from build123d import *

# Parameters (mm, degrees)
F0_W     = 11.5173384978
F0_H     = 13.0775373821
F0_W_2   = 16.1038693041
F0_H_2   = 2.9893541513
F1_DEPTH = 3


with BuildPart() as f1:
    # F0 (on Top) → F1 (new body)
    with BuildSketch(Plane.XY):
        with BuildLine():
            Line((-27.644963935, 33.9523106813), (-20.6479323776, 25.2299834391))
            ThreePointArc((-20.6479323776, 25.2299834391), (-19.752349447, 27.8264836408), (-19.4488823526, 30.5562803009))
            ThreePointArc((-19.4488823526, 30.5562803009), (-41.5954351034, 38.3068214365), (-29.1147480721, 18.4379226783))
            Line((-29.1147480721, 18.4379226783), (-36.1117796295, 27.1602499205))
            Line((-36.1117796295, 27.1602499205), (-27.644963935, 33.9523106813))
        make_face()
        with BuildLine():
            ThreePointArc((-29.1147480721, 18.4379226783), (-24.1007453474, 20.8608827061), (-20.6479323776, 25.2299834391))
            Line((-20.6479323776, 25.2299834391), (-27.644963935, 33.9523106813))
            Line((-27.644963935, 33.9523106813), (-36.1117796295, 27.1602499205))
            Line((-36.1117796295, 27.1602499205), (-29.1147480721, 18.4379226783))
        make_face()
        with BuildLine():
            Line((-19.5692731498, 6.5387686911), (-8.051934652, 9.5281228423))
            Line((-8.051934652, 9.5281228423), (-20.6479323776, 25.2299834391))
            ThreePointArc((-20.6479323776, 25.2299834391), (-24.1007453474, 20.8608827061), (-29.1147480721, 18.4379226783))
            Line((-29.1147480721, 18.4379226783), (-19.5692731498, 6.5387686911))
        make_face()
        with BuildLine():
            ThreePointArc((44.3078612119, 30.5562803009), (29.1485751221, 42.6823026363), (20.6479323776, 25.2299834391))
            Line((20.6479323776, 25.2299834391), (27.644963935, 33.9523106813))
            Line((27.644963935, 33.9523106813), (36.1117796295, 27.1602499205))
            Line((36.1117796295, 27.1602499205), (29.1147480721, 18.4379226783))
            ThreePointArc((29.1147480721, 18.4379226783), (39.6289129179, 20.8392169798), (44.3078612119, 30.5562803009))
        make_face()
        with BuildLine():
            Line((27.644963935, 33.9523106813), (20.6479323776, 25.2299834391))
            ThreePointArc((20.6479323776, 25.2299834391), (24.1007453474, 20.8608827061), (29.1147480721, 18.4379226783))
            Line((29.1147480721, 18.4379226783), (36.1117796295, 27.1602499205))
            Line((36.1117796295, 27.1602499205), (27.644963935, 33.9523106813))
        make_face()
        with BuildLine():
            Line((20.6479323776, 25.2299834391), (8.051934652, 9.5281228423))
            Line((8.051934652, 9.5281228423), (19.5692731498, 6.5387686911))
            Line((19.5692731498, 6.5387686911), (29.1147480721, 18.4379226783))
            ThreePointArc((29.1147480721, 18.4379226783), (24.1007453474, 20.8608827061), (20.6479323776, 25.2299834391))
        make_face()
        with BuildLine():
            ThreePointArc((44.3078612119, -30.5562803009), (39.6289129179, -20.8392169798), (29.1147480721, -18.4379226783))
            Line((29.1147480721, -18.4379226783), (36.1117796295, -27.1602499205))
            Line((36.1117796295, -27.1602499205), (27.644963935, -33.9523106813))
            Line((27.644963935, -33.9523106813), (20.6479323776, -25.2299834391))
            ThreePointArc((20.6479323776, -25.2299834391), (29.1485751221, -42.6823026363), (44.3078612119, -30.5562803009))
        make_face()
        with BuildLine():
            Line((36.1117796295, -27.1602499205), (29.1147480721, -18.4379226783))
            ThreePointArc((29.1147480721, -18.4379226783), (24.1007453474, -20.8608827061), (20.6479323776, -25.2299834391))
            Line((20.6479323776, -25.2299834391), (27.644963935, -33.9523106813))
            Line((27.644963935, -33.9523106813), (36.1117796295, -27.1602499205))
        make_face()
        with BuildLine():
            Line((29.1147480721, -18.4379226783), (19.5692731498, -6.5387686911))
            Line((19.5692731498, -6.5387686911), (8.051934652, -9.5281228423))
            Line((8.051934652, -9.5281228423), (20.6479323776, -25.2299834391))
            ThreePointArc((20.6479323776, -25.2299834391), (24.1007453474, -20.8608827061), (29.1147480721, -18.4379226783))
        make_face()
        with BuildLine():
            Line((-36.1117796295, -27.1602499205), (-29.1147480721, -18.4379226783))
            ThreePointArc((-29.1147480721, -18.4379226783), (-41.5954351034, -38.3068214365), (-19.4488823526, -30.5562803009))
            ThreePointArc((-19.4488823526, -30.5562803009), (-19.752349447, -27.8264836408), (-20.6479323776, -25.2299834391))
            Line((-20.6479323776, -25.2299834391), (-27.644963935, -33.9523106813))
            Line((-27.644963935, -33.9523106813), (-36.1117796295, -27.1602499205))
        make_face()
        with BuildLine():
            ThreePointArc((-20.6479323776, -25.2299834391), (-24.1007453474, -20.8608827061), (-29.1147480721, -18.4379226783))
            Line((-29.1147480721, -18.4379226783), (-36.1117796295, -27.1602499205))
            Line((-36.1117796295, -27.1602499205), (-27.644963935, -33.9523106813))
            Line((-27.644963935, -33.9523106813), (-20.6479323776, -25.2299834391))
        make_face()
        with BuildLine():
            Line((-8.051934652, -9.5281228423), (-19.5692731498, -6.5387686911))
            Line((-19.5692731498, -6.5387686911), (-29.1147480721, -18.4379226783))
            ThreePointArc((-29.1147480721, -18.4379226783), (-24.1007453474, -20.8608827061), (-20.6479323776, -25.2299834391))
            Line((-20.6479323776, -25.2299834391), (-8.051934652, -9.5281228423))
        make_face()
        with Locations((-13.8106039009, 0)):
            Rectangle(F0_W, F0_H)
        Rectangle(F0_W_2, F0_H)
        with Locations((13.8106039009, 0)):
            Rectangle(F0_W, F0_H)
        with Locations((0, -8.0334457667)):
            Rectangle(F0_W_2, F0_H_2)
        with Locations((0, 8.0334457667)):
            Rectangle(F0_W_2, F0_H_2)
        Polygon((-8.051934652, 6.5387686911), (-8.051934652, 9.5281228423), (-19.5692731498, 6.5387686911), align=None)
        Polygon((-8.051934652, -6.5387686911), (-19.5692731498, -6.5387686911), (-8.051934652, -9.5281228423), align=None)
        Polygon((8.051934652, -9.5281228423), (19.5692731498, -6.5387686911), (8.051934652, -6.5387686911), align=None)
        Polygon((19.5692731498, 6.5387686911), (8.051934652, 9.5281228423), (8.051934652, 6.5387686911), align=None)
    extrude(amount=F1_DEPTH)


solid = f1.part
Source: CAD feature listing. Evaluate the final solid. Frame: model axes, mm. A direction names the side the tool comes from. Round coordinates to 2 decimals unless told otherwise and drop trailing zeros. Loops run counter-clockwise (first coordinate to the right, second up) from the corner with the lowest first, then second, coordinate; pieces in that order, holes last.
Q1. Section C-C, the plane x = 32.5. Return loops of the section in (y, z), plus the area to 3 significant figures.
Q2. Access query for faces 4 (the face through (0, 9.528, 1)), 5 (the face through (-1, 1, 3)). Directions: +Z, -Z, +X, -X, +Y, -Y. A direction counts if a zero-diameter tool reaches every point of the face in a straight line with its end or side. Return the directions, or none.
Q3. Mould query, pull axis X, two halves, no side actions, for faces 1 (the face through (-19.569, 0, 1)), 2 (the face through (19.569, 0, 1)), 3 (the face through (0, -9.528, 1)). Classes: pulls with the +X half, pulls with the -X half, needs draft (parallel to the pull), parting line crosses it, or undercut.
Q4. Section A-A, the plane z = 2.2. Return loops of the section in (x, y), plus the area to 3 significant figures.
Q5. First-contact query: P1, Ø0.9, axis at y = 1.5, z = 1, coming from the -X side; P2, Ø5, axis at x = -20.5, y = 5.5, coming from the -Z side; P3, Ø1.5, axis at x = -3.5, z = 1.5, coming from the +Y side. Flat tips, straight axial feed; report the tip coordinate or a pass-through.
Q6. Ray query, line 1 (X direction, y = 26.5, z = 1.35); line 2 (X direction, y = 15.5, z = 2.25); line 3 (Y direction, x = -39.5, z = 0.8). Return the intervals inside material, ascending.
Q7. Section B-B, the plane y = -12. Return loops of the section in (x, z).
Q8. Section D-D, the plane x = -1. Return loops of the section in (y, z).
Solutions:
1. outline: (-42.97, 0) - (-18.14, 0) - (-18.14, 3) - (-42.97, 3) - close; (18.14, 0) - (42.97, 0) - (42.97, 3) - (18.14, 3) - close
1. area: 149 mm2
2. face 4: +Z, -Z, +Y
2. face 5: +Z, +X, -X, +Y, -Y
3. face 1: pulls with the -X half
3. face 2: pulls with the +X half
3. face 3: undercut
4. outline: (-29.11, -18.44) arc R12.43 ccw (long way) to (-20.65, -25.23) - (-8.05, -9.53) - (8.05, -9.53) - (20.65, -25.23) arc R12.43 ccw (long way) to (29.11, -18.44) - (19.57, -6.54) - (19.57, 6.54) - (29.11, 18.44) arc R12.43 ccw (long way) to (20.65, 25.23) - (8.05, 9.53) - (-8.05, 9.53) - (-20.65, 25.23) arc R12.43 ccw (long way) to (-29.11, 18.44) - (-19.57, 6.54) - (-19.57, -6.54) - close
4. area: 3,350 mm2
5. P1: stops at x = -19.57
5. P2: stops at z = 0
5. P3: stops at y = 9.53
6. line 1: x = -43.63 to -20.13, 20.13 to 43.63
6. line 2: x = -26.76 to -12.84, 12.84 to 26.76
6. line 3: y = -40.37 to -20.74, 20.74 to 40.37
7. outline: (-23.95, 0) - (-10.03, 0) - (-10.03, 3) - (-23.95, 3) - close; (10.03, 0) - (23.95, 0) - (23.95, 3) - (10.03, 3) - close
8. outline: (-9.53, 0) - (9.53, 0) - (9.53, 3) - (-9.53, 3) - close
